CAD build for the part. Positions are in the model's coordinates, mm. A direction names the side the tool comes from. Coordinates: 2 decimals unless noted, no trailing zeros. Loops run counter-clockwise (first coordinate to the right, second up) from the corner with the lowest first, then second, coordinate; pieces in that order, holes last.
1) Saw through at B-B, the plane x = -13.5. Write the cut outline in (y, z).
2) Wall check: line 1 along Z through (x, y) = (-4.5, 1); line 2 along Z through (x, y) = (-12, 7.75); line 3 along Y through (x, z) = (-6.5, 2). Give the ranges that are in metal, low to high.
3) Saw through at C-C, the plane y = 13. Give the number of separate pieces and of enclosed holes in the cut face, and give its area (3 significant figures).
4) Pin check, flat tips, straight feed: pin 1 Ø4 at (x, y) = (-4.5, 6) entering from +Z; pin 2 Ø1.5 at (x, y) = (-13, 4.5) entering from +Z; pin 3 Ø0.8 at (y, z) = (5, 4) entering from -X. Stop position of each tip, or through.
5) Saw through at A-A, the plane y = 9.5. Write the cut outline in (x, z), and give its area (3 significant figures).
6) Which spindle directions (+Z, -Z, +X, -X, +Y, -Y) get a long thin tool onto all of the face, cutting with end or side? Do faces 5 (the flat face through (0, 9, 3)), 6 (the flat face through (-5, 5, 5)), 7 (the flat face through (-15, 7, 4)). Say none if no direction does.
7) Two-plate mould, pull along Y, no slides. Class faces 1 (the flat face through (-10, 12, 6)), 2 (the flat face through (-8, 0, 2)), 3 (the flat face through (-8, 14.11, 3)), 4 (the flat face through (-15.5, 7.1, 3)): +Y half, -Y half, draft (parallel to the pull), parting line (faces both ways), or undercut.
```python
from build123d import *

# Parameters (mm, degrees)
F0_W        = 16
F0_H        = 14
F1_DEPTH    = 5
F2_W        = 1
F2_H        = 14
F3_DEPTH    = 2
F5_DEPTH    = 0.5
F6_W        = 10
F6_H        = 4
F7_DEPTH    = 3.5
F8_T4_DEPTH = 35.959416678
F10_DEPTH   = 0.11
F11_R       = 0.3
F12_DEPTH   = 2.3


# Not quite as in the source:
# - a fillet or chamfer that OpenCascade refuses, or shapes differently, is made with other operations: its cross-section is extruded or revolved along the edge and cut away or added


with BuildPart() as f1:
    # F0 (on Top) → F1 (new body)
    with BuildSketch(Plane.XY):
        with Locations((-8, 7)):
            Rectangle(F0_W, F0_H)
    extrude(amount=F1_DEPTH)

    # F2 (on face) → F3 (cut)
    with BuildSketch(Plane.XY.offset(5)):
        with Locations((-15.5, 7)):
            Rectangle(F2_W, F2_H)
    extrude(amount=-F3_DEPTH, mode=Mode.SUBTRACT)

    # F4 (on face) → F5 (cut, symmetric)
    with BuildSketch(Plane.XY.offset(5)):
        Polygon((-10, 14), (-15, 14), (-15, 0), (-10.8115321142, 0), (-10.8115321142, 8.5921764899), (-10, 9.1764843091), align=None)
    extrude(amount=F5_DEPTH, both=True, mode=Mode.SUBTRACT)

    # F6 (on face) → F7 (join)
    with BuildSketch(Plane.XY.offset(5)):
        with Locations((-5, 12)):
            Rectangle(F6_W, F6_H)
    extrude(amount=F7_DEPTH)

    # F8: chamfer of 5 x 1.5 on 1 edges, made by hand


with BuildPart() as f8_tool2:
    # F8_s3 → F8_t4 (new body)
    with BuildSketch(Plane.YZ.offset(-22.979708339)):
        Polygon((10, 3.5), (11.5, 8.5), (10, 8.5), align=None)
    extrude(amount=F8_T4_DEPTH)

    split(bisect_by=Plane.XY.offset(5), keep=Keep.TOP)


with BuildPart() as f1_1:
    add(f1.part)

    # F8_t1: cut F8_tool2
    add(f8_tool2.part, mode=Mode.SUBTRACT)

    # F9 (on face) → F10 (join)
    with BuildSketch(Plane(origin=(0, 14, 0), x_dir=(-1, 0, 0), z_dir=(0, 1, 0))):
        Polygon((15, 4.8544388264), (10, 4.8544388264), (10, 0), (16, 0), (16, 3), (16, 4.8544388264), align=None)
        Polygon((10, 4.5), (10, 4.8544388264), (10, 8.5), (0, 8.5), (0, 0), (10, 0), align=None)
    extrude(amount=F10_DEPTH)

    # F11 (on face) → F12 (cut)
    with BuildSketch(Plane(origin=(0, 14.11, 0), x_dir=(-1, 0, 0), z_dir=(0, 1, 0))):
        with Locations((1.9506971954, 7.1659904264)):
            Circle(F11_R)
        with Locations((2.8280317048, 7.026860631)):
            Circle(F11_R)
        with Locations((4.8750384645, 7.7731783739)):
            Circle(F11_R)
        with Locations((3.1497415967, 6.2874185075)):
            Circle(F11_R)
        with Locations((2.0762382736, 6.2197762835)):
            Circle(F11_R)
        with BuildLine():
            ThreePointArc((0.9178482584, 2.5111044793), (0.6178482584, 2.8111044793), (0.3178482584, 2.5111044793))
            ThreePointArc((0.3178482584, 2.5111044793), (0.6178482584, 2.2111044793), (0.9178482584, 2.5111044793))
        make_face()
        with Locations((1.2844419159, 2.2510312947)):
            Circle(F11_R)
        with Locations((2.223139369, 2.0780317048)):
            Circle(F11_R)
        with Locations((1.6878734876, 3.0424325256)):
            Circle(F11_R)
        with Locations((2.2534648226, 4.0737193912)):
            Circle(F11_R)
        with Locations((2.3235260528, 4.8911064992)):
            Circle(F11_R)
        with Locations((2.6314037386, 5.6515284814)):
            Circle(F11_R)
        with Locations((1.4768216261, 4.1250384645)):
            Circle(F11_R)
        with BuildLine():
            ThreePointArc((0.9178482584, 4.0984628722), (0.6178482584, 4.3984628722), (0.3178482584, 4.0984628722))
            ThreePointArc((0.3178482584, 4.0984628722), (0.6178482584, 3.7984628722), (0.9178482584, 4.0984628722))
        make_face()
        with Locations((0.8485789713, 3.4970383785)):
            Circle(F11_R)
        with Locations((0.8190860416, 4.816750592)):
            Circle(F11_R)
        with BuildLine():
            ThreePointArc((0.9178482584, 5.5358964019), (0.6178482584, 5.8358964019), (0.3178482584, 5.5358964019))
            ThreePointArc((0.3178482584, 5.5358964019), (0.6178482584, 5.2358964019), (0.9178482584, 5.5358964019))
        make_face()
        with Locations((1.1988501004, 6.0809853088)):
            Circle(F11_R)
        with BuildLine():
            ThreePointArc((2.736303091, 8.1066926941), (3.0010312947, 7.6655580841), (3.2657594984, 8.1066926941))
            Line((3.2657594984, 8.1066926941), (2.736303091, 8.1066926941))
        make_face()
        with BuildLine():
            ThreePointArc((2.3086588338, 7.8268786892), (2.2561014313, 7.9965022753), (2.1168444274, 8.1066926941))
            Line((2.1168444274, 8.1066926941), (1.9004732402, 8.1066926941))
            ThreePointArc((1.9004732402, 8.1066926941), (1.8390352477, 7.5794360918), (2.3086588338, 7.8268786892))
        make_face()
        with Locations((3.7924325256, 7.5621265124)):
            Circle(F11_R)
        with Locations((4.6189634766, 6.9756818416)):
            Circle(F11_R)
        with Locations((3.3696561493, 5.288646793)):
            Circle(F11_R)
        with Locations((3.1127397891, 4.6683982895)):
            Circle(F11_R)
        with Locations((3.8232160392, 5.7836191645)):
            Circle(F11_R)
        with Locations((3.0834548634, 3.9976847774)):
            Circle(F11_R)
        with Locations((3.2853335664, 3.3574042049)):
            Circle(F11_R)
        with Locations((2.8300085443, 2.5571717702)):
            Circle(F11_R)
        with Locations((3.4253850562, 1.9927631688)):
            Circle(F11_R)
        with Locations((2.0840095736, 1.2006971954)):
            Circle(F11_R)
        with Locations((3.0302237165, 1.3262382736)):
            Circle(F11_R)
        with BuildLine():
            ThreePointArc((3.4639975022, 0.5034865462), (3.1690146912, 0.7488501004), (2.8740318802, 0.5034865462))
            Line((2.8740318802, 0.5034865462), (3.4639975022, 0.5034865462))
        make_face()
        with Locations((4.0301234909, 0.8606430113)):
            Circle(F11_R)
        with Locations((4.2602388243, 2.4640656129)):
            Circle(F11_R)
        with Locations((4.9156774171, 2.3187574119)):
            Circle(F11_R)
        with Locations((6.1767839608, 2.7163808355)):
            Circle(F11_R)
        with Locations((6.6303438507, 3.211353207)):
            Circle(F11_R)
        with Locations((6.8872602109, 3.8316017105)):
            Circle(F11_R)
        with Locations((6.9165451366, 4.5023152226)):
            Circle(F11_R)
        with Locations((6.7146664336, 5.1425957951)):
            Circle(F11_R)
        with Locations((5.7397611757, 6.0359343871)):
            Circle(F11_R)
        with Locations((5.0843225829, 6.1812425881)):
            Circle(F11_R)
        with Locations((4.4187134422, 6.0936144309)):
            Circle(F11_R)
        with Locations((6.9697762835, 7.1737617264)):
            Circle(F11_R)
        with Locations((6.2206041032, 6.7167095404)):
            Circle(F11_R)
        with Locations((7.9159904264, 7.2993028046)):
            Circle(F11_R)
        with Locations((8.6122723296, 6.9872750901)):
            Circle(F11_R)
        with Locations((7.776860631, 6.4219682952)):
            Circle(F11_R)
        with Locations((6.8934514885, 6.2473411813)):
            Circle(F11_R)
        with Locations((7.3980573997, 5.600500293)):
            Circle(F11_R)
        with Locations((8.7155580841, 6.2489687053)):
            Circle(F11_R)
        with Locations((9.0350275859, 5.6900447235)):
            Circle(F11_R)
        with Locations((8.3121265124, 5.4575674744)):
            Circle(F11_R)
        with Locations((7.6895853873, 4.8336615271)):
            Circle(F11_R)
        with BuildLine():
            Line((9.4149392098, 4.8595804226), (9.4149392098, 5.1463428204))
            ThreePointArc((9.4149392098, 5.1463428204), (8.8514210287, 5.0029616215), (9.4149392098, 4.8595804226))
        make_face()
        with Locations((7.7421319101, 4.0149618731)):
            Circle(F11_R)
        with Locations((7.5510279791, 3.2171463882)):
            Circle(F11_R)
        with Locations((7.9237617264, 2.2802237165)):
            Circle(F11_R)
        with Locations((7.1332540171, 2.5111044793)):
            Circle(F11_R)
        with Locations((8.8011498996, 2.4190146912)):
            Circle(F11_R)
        with Locations((8.6861317977, 1.6665054718)):
            Circle(F11_R)
        with Locations((8.0493028046, 1.3340095736)):
            Circle(F11_R)
        with Locations((7.1719682952, 1.473139369)):
            Circle(F11_R)
        with Locations((5.7830224588, 1.6115523195)):
            Circle(F11_R)
        with Locations((4.9705388617, 1.4979712257)):
            Circle(F11_R)
        with BuildLine():
            Line((4.9246581604, 0.5034865462), (5.3252649106, 0.5034865462))
            ThreePointArc((5.3252649106, 0.5034865462), (5.1249615355, 1.0268216261), (4.9246581604, 0.5034865462))
        make_face()
        with BuildLine():
            Line((6.7005700373, 0.5034865462), (7.2973673733, 0.5034865462))
            ThreePointArc((7.2973673733, 0.5034865462), (6.9989687053, 0.8344419159), (6.7005700373, 0.5034865462))
        make_face()
        with Locations((6.2075674744, 0.9378734876)):
            Circle(F11_R)
        with Locations((6.5259310741, 1.9595710684)):
            Circle(F11_R)
        with Locations((5.5812865578, 2.4063855691)):
            Circle(F11_R)
        with Locations((4.160673016, 1.6289199655)):
            Circle(F11_R)
        with Locations((9.0539995581, 3.0424325256)):
            Circle(F11_R)
        with Locations((8.3893569887, 3.2801234909)):
            Circle(F11_R)
        with BuildLine():
            Line((9.4149392098, 3.4955470327), (9.4149392098, 3.8709517832))
            ThreePointArc((9.4149392098, 3.8709517832), (8.8809139584, 3.683249408), (9.4149392098, 3.4955470327))
        make_face()
        with Locations((8.5231783739, 4.3749615355)):
            Circle(F11_R)
        with Locations((3.694026347, 2.8247838586)):
            Circle(F11_R)
        with Locations((1.1956938542, 1.4342324575)):
            Circle(F11_R)
        with Locations((2.427445296, 3.2719955888)):
            Circle(F11_R)
        with Locations((1.6106430113, 5.2198765091)):
            Circle(F11_R)
        with Locations((1.1407076381, 6.8986527622)):
            Circle(F11_R)
        with Locations((3.8324830337, 6.7422749581)):
            Circle(F11_R)
        with Locations((5.4393006869, 6.9668999319)):
            Circle(F11_R)
        with Locations((5.9698765091, 7.6393569887)):
            Circle(F11_R)
    extrude(amount=-F12_DEPTH, mode=Mode.SUBTRACT)


solid = f1_1.part
```
Data:
1. outline: (0, 0) - (14.11, 0) - (14.11, 4.85) - (14, 4.85) - (14, 4.5) - (0, 4.5) - close
2. line 1: z = 0 to 5
2. line 2: z = 0 to 4.5
2. line 3: y = 0 to 11.81
3. separate pieces: 1
3. enclosed holes: 83
3. area: 87.4 mm2
4. pin 1: stops at z = 5
4. pin 2: stops at z = 4.5
4. pin 3: stops at x = -15
5. outline: (-16, 0) - (0, 0) - (0, 5) - (-10, 5) - (-10, 4.5) - (-15, 4.5) - (-15, 3) - (-16, 3) - close
5. area: 75.5 mm2
6. face 5: +Z, -Z, +X, +Y, -Y
6. face 6: +Z, +X, -X, -Y
6. face 7: +Z, -X, -Y
7. face 1: undercut
7. face 2: -Y half
7. face 3: +Y half
7. face 4: draft
